Design review of the part built by this model. Coordinates are the model's own, in mm. A direction names the side the tool comes from. Round coordinates to 2 decimals unless told otherwise and drop trailing zeros. Write each loop counter-clockwise with the first axis right and the second up, starting at its lowest first coordinate (ties: lowest second). Pieces come first, ordered by that corner, then holes.
from build123d import *

# Parameters (mm, degrees)
BOSS_EXTRUDE1_DEPTH             = 6.35
BOSS_EXTRUDE3_START             = -7.9375
BOSS_EXTRUDE3_DEPTH             = 22.225
CUT_EXTRUDE4_DEPTH              = 6.08
CUT_EXTRUDE4_DEPTH_BACK         = 16.875
CUT_EXTRUDE10_START             = -19.05
SKETCH16_W                      = 4.7625
SKETCH16_H                      = 4.7625
CUT_EXTRUDE10_DEPTH             = 29.091259281
CUT_EXTRUDE11_REACH             = 13.113
CUT_EXTRUDE11_DIRECTION_2_REACH = 13.113
F_2_CLEARANCE_HOLE1_D           = 2.4384
BOSS_EXTRUDE19_DEPTH            = 6.35
CUT_EXTRUDE12_DEPTH             = 4.7625
CUT_EXTRUDE12_DEPTH_BACK        = 4.7625
CUT_EXTRUDE13_DEPTH             = 3.175
CUT_EXTRUDE14_START             = 9.525
CUT_EXTRUDE14_DEPTH             = 3.175


with BuildPart() as part:
    # Sketch2 → Boss-Extrude1 (new body)
    with BuildSketch(Plane.XY):
        with BuildLine():
            Line((4.487320853, -2.38125), (4.487320853, 2.38125))
            ThreePointArc((4.487320853, 2.38125), (-5.08, 0), (4.487320853, -2.38125))
        make_face()
    extrude(amount=BOSS_EXTRUDE1_DEPTH)

    # Sketch3 → Boss-Extrude3 (add)
    with BuildSketch(Plane.XY.offset(BOSS_EXTRUDE3_START)):
        with BuildLine():
            Line((4.487320853, 2.38125), (4.487320853, -2.38125))
            Line((4.487320853, -2.38125), (7.464780529, -7.539384784))
            ThreePointArc((7.464780529, -7.539384784), (13.566062361, -13.641452925), (21.901057446, -15.875))
            Line((21.901057446, -15.875), (35.711259281, -15.875))
            ThreePointArc((35.711259281, -15.875), (41.690195135, -11.663884303), (39.7390552, -4.615890098))
            ThreePointArc((39.7390552, -4.615890098), (22.990060642, 3.300382048), (4.487320853, 2.38125))
        make_face()
    extrude(amount=BOSS_EXTRUDE3_DEPTH)

    # Sketch14 → Cut-Extrude4 (cut, two sides)
    with BuildSketch(Plane(origin=(0, 0, 0), x_dir=(1, 0, 0), z_dir=(0, 1, 0))) as cut_extrude4_sk:
        with BuildLine():
            Line((4.487320853, -6.35), (21.428093277, -12.823412845))
            ThreePointArc((21.428093277, -12.823412845), (25.327691566, -13.918413536), (29.361259281, -14.2875))
            Line((29.361259281, -14.2875), (4.487320853, -14.2875))
            Line((4.487320853, -14.2875), (4.487320853, -6.35))
        make_face()
        with BuildLine():
            Line((4.487320853, 0), (21.428093277, 6.473412845))
            ThreePointArc((21.428093277, 6.473412845), (25.327691566, 7.568413536), (29.361259281, 7.9375))
            Line((29.361259281, 7.9375), (4.487320853, 7.9375))
            Line((4.487320853, 7.9375), (4.487320853, 0))
        make_face()
    extrude(amount=CUT_EXTRUDE4_DEPTH, mode=Mode.SUBTRACT)
    extrude(cut_extrude4_sk.sketch, amount=-CUT_EXTRUDE4_DEPTH_BACK, mode=Mode.SUBTRACT)

    # Sketch16 → Cut-Extrude10 (cut, through all)
    with BuildSketch(Plane(origin=(42.061259281, 0, 0), x_dir=(0, 0, -1), z_dir=(1, 0, 0)).offset(CUT_EXTRUDE10_START)):
        with Locations((-3.175, -9.58215)):
            Rectangle(SKETCH16_W, SKETCH16_H)
    extrude(amount=-CUT_EXTRUDE10_DEPTH, mode=Mode.SUBTRACT)

    # Cut-Extrude11: up to this face of the body (flat: up to its plane)
    cut_extrude11_end = Plane(part.part.faces().sort_by_distance((15.949219939, -9.473187723, 5.55625))[0])
    # Sketch29 → Cut-Extrude11 (cut, up to the picked face)
    with BuildSketch(Plane(origin=(0, 0, 3.175), x_dir=(-1, 0, 0), z_dir=(0, 0, -1)), mode=Mode.PRIVATE) as cut_extrude11_sk1:
        Polygon((-7.269395019, -7.2009), (-23.011259281, -7.2009), (-6.432122374, -5.75041347), align=None)
    cut_extrude11_tool1 = split(extrude(cut_extrude11_sk1.sketch, amount=-CUT_EXTRUDE11_REACH, mode=Mode.PRIVATE), bisect_by=cut_extrude11_end, keep=Keep.BOTH, mode=Mode.PRIVATE)
    add(cut_extrude11_tool1.solids().sort_by_distance((12.237592, -6.717404, 3.175))[0], mode=Mode.SUBTRACT)
    # Sketch29 → Cut-Extrude11 (cut, up to the picked face)
    with BuildSketch(Plane(origin=(0, 0, 3.175), x_dir=(-1, 0, 0), z_dir=(0, 0, -1)), mode=Mode.PRIVATE) as cut_extrude11_sk2:
        with BuildLine():
            Line((-23.011259281, -11.9634), (-13.549349632, -13.63178996))
            ThreePointArc((-13.549349632, -13.63178996), (-12.324513592, -12.849454696), (-11.172481099, -11.9634))
            Line((-11.172481099, -11.9634), (-23.011259281, -11.9634))
        make_face()
    cut_extrude11_tool2 = split(extrude(cut_extrude11_sk2.sketch, amount=-CUT_EXTRUDE11_REACH, mode=Mode.PRIVATE), bisect_by=cut_extrude11_end, keep=Keep.BOTH, mode=Mode.PRIVATE)
    add(cut_extrude11_tool2.solids().sort_by_distance((15.867281, -12.523197, 3.175))[0], mode=Mode.SUBTRACT)

    # Cut-Extrude11 direction 2: up to this face of the body (flat: up to its plane)
    cut_extrude11_direction_2_end = Plane(part.part.faces().sort_by_distance((15.949219939, -9.473187723, 0.79375))[0])
    # Sketch29 → Cut-Extrude11 direction 2 (cut, up to the picked face)
    with BuildSketch(Plane(origin=(0, 0, 3.175), x_dir=(-1, 0, 0), z_dir=(0, 0, -1)), mode=Mode.PRIVATE) as cut_extrude11_direction_2_sk1:
        Polygon((-7.269395019, -7.2009), (-23.011259281, -7.2009), (-6.432122374, -5.75041347), align=None)
    cut_extrude11_direction_2_tool1 = split(extrude(cut_extrude11_direction_2_sk1.sketch, amount=CUT_EXTRUDE11_DIRECTION_2_REACH, mode=Mode.PRIVATE), bisect_by=cut_extrude11_direction_2_end, keep=Keep.BOTH, mode=Mode.PRIVATE)
    add(cut_extrude11_direction_2_tool1.solids().sort_by_distance((12.237592, -6.717404, 3.175))[0], mode=Mode.SUBTRACT)
    # Sketch29 → Cut-Extrude11 direction 2 (cut, up to the picked face)
    with BuildSketch(Plane(origin=(0, 0, 3.175), x_dir=(-1, 0, 0), z_dir=(0, 0, -1)), mode=Mode.PRIVATE) as cut_extrude11_direction_2_sk2:
        with BuildLine():
            Line((-23.011259281, -11.9634), (-13.549349632, -13.63178996))
            ThreePointArc((-13.549349632, -13.63178996), (-12.324513592, -12.849454696), (-11.172481099, -11.9634))
            Line((-11.172481099, -11.9634), (-23.011259281, -11.9634))
        make_face()
    cut_extrude11_direction_2_tool2 = split(extrude(cut_extrude11_direction_2_sk2.sketch, amount=CUT_EXTRUDE11_DIRECTION_2_REACH, mode=Mode.PRIVATE), bisect_by=cut_extrude11_direction_2_end, keep=Keep.BOTH, mode=Mode.PRIVATE)
    add(cut_extrude11_direction_2_tool2.solids().sort_by_distance((15.867281, -12.523197, 3.175))[0], mode=Mode.SUBTRACT)

    # 2 Clearance Hole1 (through all)
    with Locations(Plane.ZY.offset(-23.011259281)):
        with Locations((3.175, -9.58215)):
            Hole(F_2_CLEARANCE_HOLE1_D / 2)

    # Sketch25 → Boss-Extrude19 (add)
    with BuildSketch(Plane.XY.offset(6.35)):
        with BuildLine():
            Line((5.183826817, -3.587873106), (4.487320853, -2.38125))
            ThreePointArc((4.487320853, -2.38125), (4.086603081, -3.017627422), (3.596326817, -3.587873106))
            Line((3.596326817, -3.587873106), (5.183826817, -3.587873106))
        make_face()
        with BuildLine():
            Line((4.259998652, 2.767455779), (5.847498652, 2.767455779))
            ThreePointArc((5.847498652, 2.767455779), (5.165618018, 2.580663195), (4.487320853, 2.38125))
            ThreePointArc((4.487320853, 2.38125), (4.377920551, 2.576860812), (4.259998652, 2.767455779))
        make_face()
    extrude(amount=-BOSS_EXTRUDE19_DEPTH)

    # Sketch32 → Cut-Extrude12 (cut, two sides)
    with BuildSketch(Plane(origin=(0, 0, 3.175), x_dir=(-1, 0, 0), z_dir=(0, 0, -1))) as cut_extrude12_sk:
        with BuildLine():
            Line((-29.361259281, -15.875), (-21.901057446, -15.875))
            ThreePointArc((-21.901057446, -15.875), (-21.664551554, -15.873322074), (-21.428093277, -15.868288634))
            ThreePointArc((-21.428093277, -15.868288634), (-17.349223696, -15.24146238), (-13.549349632, -13.63178996))
            Line((-13.549349632, -13.63178996), (-16.19315137, -13.165616382))
            ThreePointArc((-16.19315137, -13.165616382), (-18.992500475, -14.004371432), (-21.901057446, -14.2875))
            Line((-21.901057446, -14.2875), (-35.711259281, -14.2875))
            ThreePointArc((-35.711259281, -14.2875), (-37.533789128, -13.924976274), (-39.078855326, -12.892596045))
            Line((-39.078855326, -12.892596045), (-40.201387342, -14.015128061))
            ThreePointArc((-40.201387342, -14.015128061), (-38.141299077, -15.391635031), (-35.711259281, -15.875))
            Line((-35.711259281, -15.875), (-29.361259281, -15.875))
        make_face()
    extrude(amount=CUT_EXTRUDE12_DEPTH, mode=Mode.SUBTRACT)
    extrude(cut_extrude12_sk.sketch, amount=-CUT_EXTRUDE12_DEPTH_BACK, mode=Mode.SUBTRACT)

    # Sketch33 → Cut-Extrude13 (cut)
    with BuildSketch(Plane(origin=(0, 0, 7.9375), x_dir=(-1, 0, 0), z_dir=(0, 0, -1))):
        with BuildLine():
            Line((-21.901057446, -15.875), (-21.901057446, -14.2875))
            Line((-21.901057446, -14.2875), (-35.711259281, -14.2875))
            ThreePointArc((-35.711259281, -14.2875), (-37.533789128, -13.924976274), (-39.078855326, -12.892596045))
            Line((-39.078855326, -12.892596045), (-40.201387342, -14.015128061))
            ThreePointArc((-40.201387342, -14.015128061), (-38.141299077, -15.391635031), (-35.711259281, -15.875))
            Line((-35.711259281, -15.875), (-21.901057446, -15.875))
        make_face()
    extrude(amount=-CUT_EXTRUDE13_DEPTH, mode=Mode.SUBTRACT)

    # Sketch33_2 → Cut-Extrude14 (cut)
    with BuildSketch(Plane(origin=(0, 0, 7.9375), x_dir=(-1, 0, 0), z_dir=(0, 0, -1)).offset(CUT_EXTRUDE14_START)):
        with BuildLine():
            Line((-35.711259281, -15.875), (-21.901057446, -15.875))
            Line((-21.901057446, -15.875), (-21.901057446, -14.2875))
            Line((-21.901057446, -14.2875), (-35.711259281, -14.2875))
            ThreePointArc((-35.711259281, -14.2875), (-37.533789128, -13.924976274), (-39.078855326, -12.892596045))
            Line((-39.078855326, -12.892596045), (-40.201387342, -14.015128061))
            ThreePointArc((-40.201387342, -14.015128061), (-38.141299077, -15.391635031), (-35.711259281, -15.875))
        make_face()
    extrude(amount=CUT_EXTRUDE14_DEPTH, mode=Mode.SUBTRACT)


solid = part.part
1) Add section B-B on x = 20. State the section outline as (y, z) points.
2) For faces 4 (the face through (14.838, -6.486, 3.208)), 5 (the face through (29, -14.288, 3)), 6 (the face through (37.51, -13.935, 3.286)), list the 3-axis set-ups (+Z, -Z, +X, -X, +Y, -Y) from which the entire face can be reached by the end or side of a thin tool; tool diameter is ignored.
3) For P1, Ø12, axis at x = 14.5, y = -4, coming from the +Z side; P2, Ø3, axis at x = 34, z = 5.5, coming from the -Y side; P3, Ø8.5, axis at x = 11.5, y = -11, coming from the +Z side, all flat-tipped, find the tip position at first contact; note any pin that passes through.
4) For line 1 along Z through (x, y) = (3, -1.75); line 2 along Z through (x, y) = (29, -7.25); line 3 along Z through (x, y) = (21, -11.5), list the stretches that pass through material, from the lowest coordinate up.
5) The part is to be moulded in two halves that separate along Y. For faces 1 (the face through (15, -10, 5.556)), 2 (the face through (14.72, -3.57, -3.91)), 3 (the face through (18.952, -13.996, 3.242)), say which applies: pulls with the +Y half, pulls with the -Y half, needs draft (parallel to the pull), parting line crosses it, or undercut.
Computed:
1. outline: (-15.77, -5.93) - (3.77, -5.93) - (3.77, 12.28) - (-15.77, 12.28) - (-15.77, 7.94) - (-14.17, 7.94) - (-14.17, -1.59) - (-15.77, -1.59) - close; hole (-12.49, 0.79) - (-6.94, 0.79) - (-6.94, 5.56) - (-12.49, 5.56) - close
2. face 4: -X
2. face 5: +X, -Y
2. face 6: -Y
3. P1: stops at z = 12.47
3. P2: stops at y = -14.29
3. P3: stops at z = 10.65
4. line 1: z = 0 to 6.35
4. line 2: z = -7.93 to 14.28
4. line 3: z = -6.31 to 0.79, 5.56 to 12.66
5. face 1: undercut
5. face 2: needs draft
5. face 3: pulls with the -Y half
